Can you work these out from the model? Positions are in its coordinate system, mm. Coordinates: 2 decimals unless noted, no trailing zeros. Order: outer loops, then holes, each group sorted by start corner. A loop starts at its lowest first (then second) coordinate and runs counter-clockwise, first axis right, second up. Notation, with made-up numbers: (24.25, 19) -> (47.25, 19) arc R21 ccw to (47.25, 36) -> close; hole circle Ø10 at (-25, 35). An arc over 180 degrees is marked (long way). Answer as CSV lines item,"result".
from build123d import *

# Parameters (mm, degrees)
F0_R     = 12.7
F1_DEPTH = 457.2
F2_R     = 6.35
F3_DEPTH = 12.7


# Not quite as in the source:
# - a fillet or chamfer that OpenCascade refuses, or shapes differently, is made with other operations: its cross-section is extruded or revolved along the edge and cut away or added


with BuildPart() as f1:
    # F0 (on Right) → F1 (new body)
    with BuildSketch(Plane.YZ):
        Circle(F0_R)
    extrude(amount=F1_DEPTH)

    # F2 (on Top) → F3 (cut, symmetric)
    with BuildSketch(Plane.XY):
        with Locations((9.525, 0)):
            Circle(F2_R)
    extrude(amount=F3_DEPTH, both=True, mode=Mode.SUBTRACT)

    # F4: fillet of radius 5.08 on 1 edges, made by hand

    # F4_s1 → F4_t2 (revolve, cut)
    with BuildSketch(Plane.XY):
        with BuildLine():
            ThreePointArc((5.08, 12.7), (1.4878975516, 11.2121024484), (0, 7.62))
            Line((0, 7.62), (0, 12.7))
            Line((0, 12.7), (5.08, 12.7))
        make_face()
    revolve(axis=Axis((0, 0, 0), (1, 0, 0)), mode=Mode.SUBTRACT)


solid = f1.part
Q1. Imagine slicing it at B-B (x = 35). List the corners of the cut face in (y, z) for me.
Solution:
outline,"circle Ø25.4 at (0, 0)"
Q2. We'd pull the mould along Y, two halves only. Please class faces 1 (the cylindrical face through (227.98, -2.75, -12.4)), 2 (the cylindrical face through (12.939, 5.354, 0.178)), 3 (the flat face through (457.2, 0, 0)): pulls with the +Y half, pulls with the -Y half, needs draft (parallel to the pull), parting line crosses it, or undercut.
Solution:
face 1,"parting line crosses it"
face 2,"undercut"
face 3,"needs draft"
Q3. For P1, Ø1.5, axis at x = 107.5, y = -3, coming from the -Z side; P2, Ø1, axis at x = 285.5, z = 8, coming from the -Y side; P3, Ø5, axis at x = 343.5, z = -5.5, coming from the +Y side, each with a flat end and sliding along its axis, tell me the tip position at first contact or that it passes through.
Solution:
P1,"z = -12.5"
P2,"y = -10.25"
P3,"y = 12.34"
Q4. Imagine slicing it at A-A (y = 0). List the corners of the cut face in (x, z) for me (3 decimals).
Solution:
outline,"(0, -7.62) arc R5.08 ccw to (3.175, -12.329) -> (3.175, 12.329) arc R5.08 ccw to (0, 7.62) -> close; (15.875, -12.7) -> (457.2, -12.7) -> (457.2, 12.7) -> (15.875, 12.7) -> close"
Q5. If I drill on line 1 (X direction, y = 0, z = -6.5) (3 decimals); line 2 (Z direction, x = 321.5, y = 2.75); line 3 (Z direction, x = 71, y = -3), over which ranges is the centre line in solid material (lowest first)?
Solution:
line 1,"0 to 3.175, 15.875 to 457.2"
line 2,"-12.4 to 12.4"
line 3,"-12.34 to 12.34"
